CAD build for the part. Positions are in the model's coordinates, mm. Face numbers are marked on the shaded views. A direction names the side the tool comes from. Coordinates: 2 decimals unless noted, no trailing zeros. Loops run counter-clockwise (first coordinate to the right, second up) from the corner with the lowest first, then second, coordinate; pieces in that order, holes last. Notation, with made-up numbers: (3.5, 77.25) - (61.5, 77.25) arc R29 cw to (61.5, 115.25) - close; hole circle Ø3 at (6.5, 59.25). An arc over 180 degrees is marked (long way). Put each result on its own line as item: value.
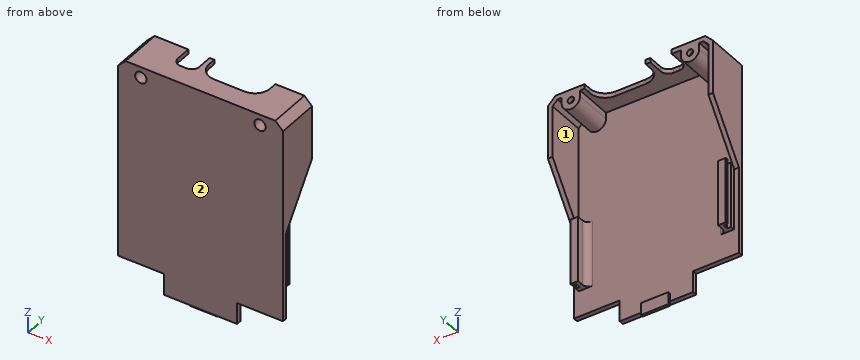
```python
from build123d import *

# Parameters (mm, degrees)
CROQUIS1_R                 = 3.75
SALIENTE_EXTRUIR1_DEPTH    = 3
SALIENTE_EXTRUIR5_START    = -17
SALIENTE_EXTRUIR5_DEPTH    = 43
SALIENTE_EXTRUIR3_DEPTH    = 3
CROQUIS4_R                 = 3.75
SALIENTE_EXTRUIR4_DEPTH    = 25
SALIENTE_EXTRUIR7_START    = -3
CROQUIS8_R                 = 3.75
CROQUIS8_R_2               = 2.1
SALIENTE_EXTRUIR7_DEPTH    = 3
CROQUIS7_W                 = 18
CROQUIS7_H                 = 8
SALIENTE_EXTRUIR6_DEPTH    = 1.8
CORTAR_EXTRUIR1_DEPTH      = 161.937876213
CORTAR_EXTRUIR1_DEPTH_BACK = 10


with BuildPart() as part:
    # Croquis1 → Saliente-Extruir1 (new body)
    with BuildSketch(Plane(origin=(0, 0, 0), x_dir=(1, 0, 0), z_dir=(0, 1, 0))):
        Polygon((-24, 60), (24, 60), (24, 46), (54, 46), (54, -81), (49, -86), (-49, -86), (-54, -81), (-54, 46), (-24, 46), align=None)
        with Locations(Location((-39, -79, 0), (0, 0, 270))):
            Circle(CROQUIS1_R, mode=Mode.SUBTRACT)
        with Locations(Location((39, -79, 0), (0, 0, 90))):
            Circle(CROQUIS1_R, mode=Mode.SUBTRACT)
    extrude(amount=SALIENTE_EXTRUIR1_DEPTH)

    # Croquis6 → Saliente-Extruir5 (add)
    with BuildSketch(Plane(origin=(0, 0, -46), x_dir=(-1, 0, 0), z_dir=(0, 0, -1)).offset(SALIENTE_EXTRUIR5_START)):
        with BuildLine():
            Line((50.8, 3), (50.8, 5.85))
            Line((50.8, 5.85), (48.2, 5.85))
            Line((48.2, 5.85), (48.2, 9.15))
            Line((48.2, 9.15), (50.8, 9.15))
            Line((50.8, 9.15), (50.8, 11))
            Line((50.8, 11), (45.8, 11))
            Line((45.8, 11), (45.8, 7))
            ThreePointArc((45.8, 7), (44.628427125, 4.171572875), (41.8, 3))
            Line((41.8, 3), (47.8, 3))
            Line((47.8, 3), (50.8, 3))
        make_face()
    saliente_extruir5 = extrude(amount=-SALIENTE_EXTRUIR5_DEPTH)

    # Croquis3 → Saliente-Extruir3 (add)
    with BuildSketch(Plane.ZY.offset(54)):
        Polygon((11, 3), (46, 28), (79.207391253, 28), (79.207391253, 3), align=None)
    saliente_extruir3 = extrude(amount=-SALIENTE_EXTRUIR3_DEPTH)

    # Croquis4 → Saliente-Extruir4 (add)
    with BuildSketch(Plane(origin=(0, 3, 0), x_dir=(1, 0, 0), z_dir=(0, 1, 0))):
        with BuildLine():
            Line((-51, -79.207391253), (-54, -79.207391253))
            Line((-54, -79.207391253), (-54, -81))
            Line((-54, -81), (-49, -86))
            Line((-49, -86), (0, -86))
            Line((0, -86), (0, -83))
            Line((0, -83), (-33, -83))
            Line((-33, -83), (-33, -79))
            ThreePointArc((-33, -79), (-39, -73), (-45, -79))
            Line((-45, -79), (-45, -83))
            Line((-45, -83), (-47.757359313, -83))
            Line((-47.757359313, -83), (-51, -79.757359313))
            Line((-51, -79.757359313), (-51, -79.207391253))
        make_face()
        with Locations((-39, -79)):
            Circle(CROQUIS4_R, mode=Mode.SUBTRACT)
    saliente_extruir4 = extrude(amount=SALIENTE_EXTRUIR4_DEPTH)

    # Croquis8 → Saliente-Extruir7 (add)
    with BuildSketch(Plane(origin=(0, 28, 0), x_dir=(1, 0, 0), z_dir=(0, 1, 0)).offset(SALIENTE_EXTRUIR7_START)):
        with Locations(Location((-39, -79, 0), (0, 0, 270))):
            Circle(CROQUIS8_R)
        with Locations(Location((-39, -79, 0), (0, 0, 270))):
            Circle(CROQUIS8_R_2, mode=Mode.SUBTRACT)
    saliente_extruir7 = extrude(amount=SALIENTE_EXTRUIR7_DEPTH)

    # Simetría1: Saliente-Extruir5, Saliente-Extruir3, Saliente-Extruir4, Saliente-Extruir7 across plane
    add(saliente_extruir5.mirror(Plane(origin=(0, 0, 0), x_dir=(0, 0, 1), z_dir=(1, 0, 0))))
    add(saliente_extruir3.mirror(Plane(origin=(0, 0, 0), x_dir=(0, 0, 1), z_dir=(1, 0, 0))))
    add(saliente_extruir4.mirror(Plane(origin=(0, 0, 0), x_dir=(0, 0, 1), z_dir=(1, 0, 0))))
    add(saliente_extruir7.mirror(Plane(origin=(0, 0, 0), x_dir=(0, 0, 1), z_dir=(1, 0, 0))))

    # Croquis7 → Saliente-Extruir6 (add)
    with BuildSketch(Plane(origin=(0, 3, 0), x_dir=(1, 0, 0), z_dir=(0, 1, 0))):
        with Locations((0, 59)):
            Rectangle(CROQUIS7_W, CROQUIS7_H)
    extrude(amount=SALIENTE_EXTRUIR6_DEPTH)

    # Croquis9 → Cortar-Extruir1 (cut, two sides: drawn at the far end of the back side and taken through both)
    with BuildSketch(Plane.XY.offset(86).offset(-CORTAR_EXTRUIR1_DEPTH_BACK)):
        with BuildLine():
            Line((30, 28), (-10, 28))
            Line((-10, 28), (-10, 23))
            ThreePointArc((-10, 23), (-7.071067812, 15.928932188), (0, 13))
            Line((0, 13), (20, 13))
            ThreePointArc((20, 13), (27.071067812, 15.928932188), (30, 23))
            Line((30, 23), (30, 28))
        make_face()
        with BuildLine():
            Line((-13, 18), (-13, 28))
            Line((-13, 28), (-27, 28))
            Line((-27, 28), (-27, 18))
            ThreePointArc((-27, 18), (-25.535533906, 14.464466094), (-22, 13))
            Line((-22, 13), (-18, 13))
            ThreePointArc((-18, 13), (-14.464466094, 14.464466094), (-13, 18))
        make_face()
    extrude(amount=CORTAR_EXTRUIR1_DEPTH + CORTAR_EXTRUIR1_DEPTH_BACK, mode=Mode.SUBTRACT)


solid = part.part
```
Q1. Tool access for the marked faces 1 and 2: list every direction of +Z, -Z, +X, -X, +Y, -Y with a clear straight run to the whole face (end or side of a thin tool).
Determined:
face 1: -Z, +Y
face 2: +Z, -Z, +X, -X, -Y
Q2. Pin check, flat tips, straight feed: pin 1 Ø8 at (y, z) = (13, -22.5) entering from +X; pin 2 Ø2 at (x, y) = (46, 10.5) entering from -Z; pin 3 Ø5.5 at (x, z) = (49, -14.5) entering from +Y. Stop position of each tip, or through.
Determined:
pin 1: x = 50.8
pin 2: z = -29
pin 3: y = 11
Q3. Slice it at C-C, the plane x = 17. Give the cut face in (y, z).
Determined:
outline: (0, -60) - (3, -60) - (3, 83) - (13, 83) - (13, 86) - (0, 86) - close
Q4. Slice it at A-A, the plane z = -9. Give the cut face in (x, y).
Determined:
outline: (-54, 0) - (54, 0) - (54, 3) - (50.8, 3) - (50.8, 5.85) - (48.2, 5.85) - (48.2, 9.15) - (50.8, 9.15) - (50.8, 11) - (45.8, 11) - (45.8, 7) arc R4 cw to (41.8, 3) - (-41.8, 3) arc R4 cw to (-45.8, 7) - (-45.8, 11) - (-50.8, 11) - (-50.8, 9.15) - (-48.2, 9.15) - (-48.2, 5.85) - (-50.8, 5.85) - (-50.8, 3) - (-54, 3) - close
Q5. Slice it at D-D, the plane z = 40.5. Give the cut face in (x, y), then the cut area to 3 significant figures.
Determined:
outline: (-54, 0) - (54, 0) - (54, 24.07) - (51, 24.07) - (51, 3) - (-51, 3) - (-51, 24.07) - (-54, 24.07) - close
area: 450 mm2
Q6. Slice it at B-B, the plane x = 39. Give the cut face in (y, z).
Determined:
outline: (0, -46) - (3, -46) - (3, 73) - (28, 73) - (28, 76.9) - (25, 76.9) - (25, 75.25) - (0, 75.25) - close; (0, 82.75) - (25, 82.75) - (25, 81.1) - (28, 81.1) - (28, 86) - (0, 86) - close
Q7. Wall check: L1, parallel to X at y = 26.75, z = 79; L2, parallel to X at y = 14.5, z = 79; L3, parallel to Z at x = 39, y = 18. Give the ranges that are in metal, low to high. Write a range as from..to.
Determined:
L1: -54..-51, -45..-41.1, -36.9..-33, 33..36.9, 41.1..45, 51..54
L2: -54..-51, -45..-42.75, -35.25..-33, 33..35.25, 42.75..45, 51..54
L3: 73..75.25, 82.75..86
